CAD build for the part. Positions are in the model's coordinates, mm. Face numbers are marked on the shaded views. A direction names the side the tool comes from. Give positions to 0.01 mm unless a question says otherwise; leave off trailing zeros. Loops run counter-clockwise (first coordinate to the right, second up) from the corner with the lowest first, then second, coordinate; pieces in that order, holes last. Notation, with made-up numbers: M -40,53.5 L 19,53.5 A19 cw 19,64.5 Z; hole C 12.25,-13 d3. An arc over 180 degrees is marked long. Answer as CSV lines item,"result".
```python
from build123d import *

# Parameters (mm, degrees)
F4_DEPTH = 2.286


# Not quite as in the source:
# - a feature names something its author has since deleted; it is built from what else it names


with BuildPart() as f2:
    # F0 (on Top) → F2 (revolve)
    with BuildSketch(Plane.XY):
        Polygon((2.4690357124, -1.7526), (15.875, -1.7526), (15.875, 0), (0, 0), (0, -3.8989), align=None)
    revolve(axis=Axis((4.9627271947, 0, 0), (1, 0, 0)))

    # F3 (on face) → F4 (cut)
    with BuildSketch(Plane(origin=(0, 0, 0), x_dir=(0, -1, 0), z_dir=(-1, 0, 0))):
        Polygon((0.5728397202, 0.9921875), (-0.5728397202, 0.9921875), (-1.1456794404, 0), (-0.5728397202, -0.9921875), (0.5728397202, -0.9921875), (1.1456794404, 0), align=None)
    extrude(amount=-F4_DEPTH, mode=Mode.SUBTRACT)


solid = f2.part
```
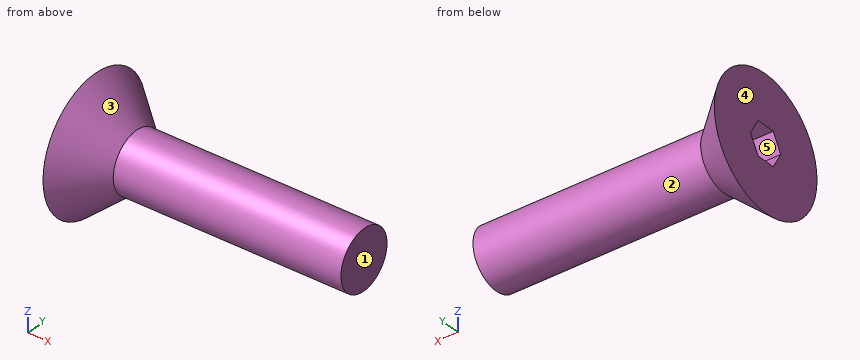
Q1. Cut at A-A (y = 0). Write the cut outline in (x, z) (3 decimals).
Solution:
outline,"M 0,-3.899 L 2.469,-1.753 L 15.875,-1.753 L 15.875,1.753 L 2.469,1.753 L 0,3.899 L 0,0.992 L 2.286,0.992 L 2.286,-0.992 L 0,-0.992 Z"
Q2. Mould opens along Y. For the marked faces 3, 4 and 5 say: released by +Y, released by -Y, zero draft, split by the parting line, or undercut.
Solution:
face 3,"split by the parting line"
face 4,"zero draft"
face 5,"undercut"
Q3. Cut at B-B (x = 8.5). Write the cut outline in (y, z), and give its area (3 significant figures).
Solution:
outline,"C 0,0 d3.51"
area,"9.65 mm²"
Q4. Pin check, flat tips, straight feed: P1, Ø0.9, axis at x = 1, y = 0, coming from the +Z side; P2, Ø0.6, axis at x = 1, y = 0.5, coming from the -Z side. Stop position of each tip, or through.
Solution:
P1,"stops at z = 3.42"
P2,"stops at z = -3.26"
Q5. Wall check: line 1 (X direction, y = -1.25, z = 2); line 2 (X direction, y = 1.5, z = 2.5); line 3 (Z direction, x = 4.5, y = -1.5). Give the ranges that are in metal, low to high. Write a range as [from, to].
Solution:
line 1,"x = [0, 1.77]"
line 2,"x = [0, 1.13]"
line 3,"z = [-0.91, 0.91]"
Q6. Which spindle directions (+Z, -Z, +X, -X, +Y, -Y) get a long thin tool onto all of the face, cutting with end or side? Do the marked faces 1 and 2. Say none if no direction does.
Solution:
face 1,"+Z, -Z, +X, +Y, -Y"
face 2,"+X"
